Part model, mm, in its own coordinate system. A direction names the side the tool comes from. Give positions to 0.01 mm unless a question says otherwise; leave off trailing zeros. Order: outer loops, then holes, each group sorted by start corner. A loop starts at its lowest first (then second) coordinate and runs counter-clockwise, first axis right, second up. Notation, with made-up numbers: (-38.5, 23) -> (-5.5, 23) arc R18 cw to (-5.5, 44) -> close; hole circle Ø4 at (64, 85.25). An arc over 180 degrees is marked (long way). Write item = value, one per line. Start each with the question number.
(1) Saw through at C-C, the plane x = 16. List the corners of the cut face in (y, z), then the cut area to 3 significant figures.
(2) Saw through at A-A, the plane x = -3.7. State how many separate pieces and enclosed holes the cut face has, then the cut area to 3 significant figures.
(3) Which spindle directions (+Z, -Z, +X, -X, +Y, -Y) get a long thin tool onto all of the face, cutting with end or side? Do faces 5 (the flat face through (-4, -2.5, 1)), 6 (the cylindrical face through (-2.74, -1.08, 4.88)). Say none if no direction does.
(4) Two-plate mould, pull along X, no slides. Class faces 1 (the cylindrical face through (-4.344, -2.042, -3.131)), 2 (the flat face through (0, 3.3, 0.1)), 3 (the cylindrical face through (-4.324, -3.733, -0.259)), 4 (the cylindrical face through (10, -3, 0)): pulls with the +X half, pulls with the -X half, needs draft (parallel to the pull), parting line crosses it, or undercut.
(5) Probe line 1 along X through (y, z) = (4.35, 0) (3 decimals); line 2 along Z through (x, y) = (2.25, 0); line 3 along Z through (x, y) = (-3.7, 4.15) (3 decimals). List the from-to ranges inside material, lowest first. Write a range as from..to.
(6) Flat gauge pins, fed straight in: pin 1 (5 mm diameter, centred on x = 5, y = 3, fed in from +Z); pin 2 (6 mm diameter, centred on x = 2, y = 2.5, fed in from -Z); pin 3 (1.6 mm diameter, centred on x = -3.7, z = 0, fed in from -Y); pin 4 (3 mm diameter, centred on x = 4.5, y = 2, fed in from -Z). Where does each tip first touch, or does it go through?
Autodesk Inventor part; units mm, degrees
ref_plane "Work Plane1" through (10, 0, 0) normal (0, 0.5, 0.866) x (1, 0, 0)
ref_plane "YZ Plane" through (0, 0, 0) normal (1, 0, 0) x (0, 1, 0)
ref_plane "XZ Plane" through (0, 0, 0) normal (0, 1, 0) x (-1, 0, 0)
sketch "Sketch1" plane through (0, 0, 0) normal (0, 0, 1) x (1, 0, 0)
  line L0 (-1.3333, 0) -> (20, 0)
  line L1 (20, 0) -> (20, 3)
  line L2 (20, 3) -> (0, 3)
  line L3 (0, 3) -> (0, 5)
  line L4 (0, 5) -> (-6, 5)
  line L5 (-6, 5) -> (-6, 2.8868)
  line L6 (-6, 2.8868) -> (-3, 2.8868)
  line L7 (-3, 2.8868) -> (-1.3333, 0)
  line L8 (-11.2, 0) -> (25.2, 0)
  line L9 (0, -1) -> (0, 6)
  dimension "d3" = 6
  dimension "d4" = 3
  dimension "d5" = 60
  dimension "d6" = 6
  dimension "d8" = 5.7735
  dimension "d9" = 10
  dimension "d31" = 20
revolve "Body" add sketch "Sketch1" angle 360 about axis through (-1.3333, 0, 0) along (1, 0, 0)
sketch "Sketch2" plane through (-6, 0, 0) normal (-1, 0, 0) x (0, 0, 1)
  circle A0 centre (0, 0) radius 2.8868
  line L0 (0, -7) -> (0, 7)
  line L1 (-7, 0) -> (7, 0)
  line L2 (2.8868, 0) -> (1.4434, -2.5)
  line L3 (1.4434, -2.5) -> (-1.4434, -2.5)
  line L4 (-1.4434, -2.5) -> (-2.8868, 0)
  line L5 (-2.8868, 0) -> (-1.4434, 2.5)
  line L6 (-1.4434, 2.5) -> (1.4434, 2.5)
  line L7 (1.4434, 2.5) -> (2.8868, 0)
extrude "Slot" add sketch "Sketch2" against normal up to next contours L7 A0 | A0 L2 | L6 L0 A0 | A0 L0 L3 | L0 L6 A0 | A0 L3 L0 | L4 A0 | A0 L5
sketch "Sketch3" plane through (-6, 0, 0) normal (-1, 0, 0) x (0, 0, 1)
  circle A0 centre (0, 0) radius 5
  line L0 (-1.4434, 2.5) -> (1.4434, 2.5)
  circle A1 centre (0, 0) radius 2.5166
  point P0 (-0.2887, 2.5)
  point P1 (0.2887, 2.5)
  dimension "d23" = 0.5774
extrude "Overcut" cut sketch "Sketch3" against normal blind 3 contours A1 L0 | L0 A1
sketch "Sketch4" plane through (0, 0, 0) normal (0, 1, 0) x (-1, 0, 0)
  line L0 (0, 5) -> (0, -5)
  line L1 (7.2, 0) -> (-1.2, 0)
  circle A0 centre (3.7, 0) radius 0.675
  line L2 (6, 5) -> (6, -5)
  point P0 (0, 0)
  dimension "d13" = 1.35
  dimension "d14" = 2.3
extrude "Hole" cut sketch "Sketch4" along normal through all both and the other way through all
pattern_circular "Holes" count 3 over 360 about axis through (10, 0, 0) along (1, 0, 0) of "Hole"
chamfer "Chamfer1" distance 0.6 angle 45 1 edges at (-6, -5, 0) measured on face at (-3.2045, -4.6671, -1.794)
thread "Thread"
chamfer "Chamfer2" distance 0.6135 distance2 0.6135 1 edges at (20, -3, 0) measured on face at (20, 1.0659, 1.0214)
ref_plane "Work Plane1" through (10, 0, 0) normal (0, 0.5, 0.866) x (1, 0, 0)
equation "\"d3\" = KOH"
equation "\"d4\" = STI"
equation "\"d6\" = GD"
equation "\"d8\" = 1.1547 * SW"
equation "\"d9\" = KOD"
equation "\"d31\" = NLG"
equation "\"d23\" = 0.11547 * SW"
equation "\"d24\" = STI"
equation "\"d13\" = BOR"
equation "\"d14\" = DIST"
equation "\"d17\" = PHH"
equation "\"d32\" = PHH"
equation "\"d19\" = GEL"
equation "\"d21\" = -0.5 * SPD + 0.5 * GD"
equation "\"d22\" = GUL"
equation "\"GD\" = NND"
equation "\"NLG\" = 20"
equation "\"GEL\" = 18.7731"
equation "\"KOD\" = 10"
equation "\"KOH\" = 6"
equation "\"GUL\" = 0.61345 * PTC"
equation "\"SW\" = 5"
equation "\"STI\" = 3"
equation "\"DIST\" = 2.3"
equation "\"BOR\" = 1.35"
equation "\"PHH\" = 0.6"
equation "\"SPD\" = 4.7731"
equation "\"PTC\" = 1"
equation "\"THREADDIA\" = 6"
equation "\"TOA\" = 30deg"
equation "\"BDM\" = NND"
equation "\"NND\" = 6"
equation "\"E0\" = 1.155 * SW"
equation "\"GAL\" = 0.61345 * PTC"
equation "\"GD1\" = THREADDIA - 1.2269 * PTC"
properties part number "ANSI B18.3.1M - M6x1 x 20" material "Steel, Mild"
Results list:
q1.outline = circle Ø6 at (0, 0)
q1.area = 28.3 mm^2
q2.separate_pieces = 6
q2.enclosed_holes = 0
q2.area = 36.8 mm^2
q3.face_5 = -X
q3.face_6 = +X, -X
q4.face_1 = undercut
q4.face_2 = pulls with the +X half
q4.face_3 = undercut
q4.face_4 = needs draft
q5.line_1 = -6..-4.375, -3.025..0
q5.line_2 = -3..3
q5.line_3 = -2.789..-0.675, 0.675..2.789
q6.pin_1 = 2.96
q6.pin_2 = -4.99
q6.pin_3 = -5
q6.pin_4 = -2.96
